Part model, mm, in its own coordinate system. A direction names the side the tool comes from. Round coordinates to 2 decimals unless told otherwise and drop trailing zeros. Loops run counter-clockwise (first coordinate to the right, second up) from the corner with the lowest first, then second, coordinate; pieces in that order, holes last. Notation, with made-up numbers: (4, 83) - (10, 83) arc R28 cw to (10, 103) - close; hole circle Ø4 at (-10, -18). An arc over 180 degrees is marked (long way). Write each question's results on one line, items separated by ' | '. Start each with the question number.
(1) Mould opens along X. For faces 4 (the face through (80.25, 2, -79)), 5 (the face through (58, 2, 80)), 6 (the face through (138.03, 2.18, -40.276)), 7 (the face through (46.263, 2, 0)) say: released by +X, released by -X, zero draft, split by the parting line, or undercut.
(2) Drill centre lines: L1, parallel to Z at x = 36, y = 1.55; L2, parallel to X at y = 2.9, z = -15; L3, parallel to Z at x = 105, y = 1.1. Where is each one in solid material? Low to high.
(3) Tool access for faces 1 (the face through (69, 2, 6)), 2 (the face through (153.27, 2.18, 57.43)), 3 (the face through (102, 2, -80)): list every direction of +Z, -Z, +X, -X, +Y, -Y with a clear straight run to the whole face (end or side of a thin tool).
(4) Cut at A-A, the plane x = 39. List the corners of the cut face in (y, z).
(5) Cut at B-B, the plane x = 112.5. List the corners of the cut face in (y, z), then the cut area to 3 significant figures.
(6) Flat gauge pins, fed straight in: P1, Ø2, axis at x = 49, y = 1.5, coming from the +Z side; P2, Ø1.3, axis at x = 10.5, y = 3, coming from the -Z side; P3, Ø1.5, axis at y = 2.5, z = -51.5, coming from the +X side. Where does each tip first touch, or does it go through?
(7) Cut at C-C, the plane y = 0.8. Give the number of separate pieces and of enclosed holes in the cut face, then the cut area to 3 significant figures.
from build123d import *

# Parameters (mm, degrees)
BOSS_EXTRUDE1_DEPTH = 4.3
CUT_EXTRUDE1_DEPTH  = 4.5
FILLET1_R           = 2
CUT_EXTRUDE2_DEPTH  = 10
SKETCH8_R           = 1.5
CUT_EXTRUDE3_DEPTH  = 10
SKETCH9_R           = 1.5
CUT_EXTRUDE4_DEPTH  = 10
CUT_EXTRUDE5_DEPTH  = 10
SKETCH11_R          = 1.5
CUT_EXTRUDE6_DEPTH  = 10
SKETCH12_R          = 1.5
CUT_EXTRUDE7_DEPTH  = 10
SKETCH7_R           = 1.5
SKETCH7_W           = 11
SKETCH7_H           = 3
CUT_EXTRUDE8_DEPTH  = 9
CUT_EXTRUDE9_DEPTH  = 10
SKETCH14_R          = 1.5
CUT_EXTRUDE10_DEPTH = 10
SKETCH15_W          = 5
SKETCH15_H          = 14
CUT_EXTRUDE11_DEPTH = 10
SKETCH16_R          = 1.5
CUT_EXTRUDE12_DEPTH = 10
SKETCH18_R          = 1.5
SKETCH18_W          = 28.4
SKETCH18_H          = 4
CUT_EXTRUDE13_DEPTH = 10


with BuildPart() as part:
    # Sketch2 → Boss-Extrude1 (new body)
    with BuildSketch(Plane(origin=(0, 0, 0), x_dir=(1, 0, 0), z_dir=(0, 1, 0))):
        Polygon((0, 0), (0, 65), (58, 65), (58, 95), (102, 95), (102, 65), (160, 65), (160, 0), align=None)
    extrude(amount=BOSS_EXTRUDE1_DEPTH)

    # Mirror1: part across plane


with BuildPart() as part_1:
    add(part.part)
    add(part.part.mirror(Plane(origin=(0, 4.3, 0), x_dir=(1, 0, 0), z_dir=(0, 0, -1))))

    # Sketch3 → Cut-Extrude1 (cut)
    with BuildSketch(Plane(origin=(0, 4.3, 0), x_dir=(1, 0, 0), z_dir=(0, 1, 0))):
        Polygon((160, 61.8), (160, -61.8), (157.155555556, -61.8), (120, -20), (80.012594795, 0), (80.012594795, 20), (120.012594795, 20), (157.156451185, 61.8), align=None)
    extrude(amount=-CUT_EXTRUDE1_DEPTH, mode=Mode.SUBTRACT)

    # Fillet1
    fillet1_edges = [part_1.edges().sort_by_distance(p)[0] for p in [
        (157.156451185, 2.15, -61.8),
        (157.155555556, 2.15, 61.8),
    ]]
    fillet(fillet1_edges, radius=FILLET1_R)

    # Sketch6 → Cut-Extrude2 (cut)
    with BuildSketch(Plane(origin=(0, 4.3, 0), x_dir=(1, 0, 0), z_dir=(0, 1, 0))):
        Polygon((9, -61.8), (49, -61.8), (49, -44.8), (43, -44.8), (43, -30.841820122), (15, -30.841820122), (15, -44.8), (9, -44.8), align=None)
        Polygon((9, 44.8), (15, 44.8), (15, 30.841820122), (43, 30.841820122), (43, 44.8), (49, 44.8), (49, 61.8), (9, 61.8), align=None)
    extrude(amount=-CUT_EXTRUDE2_DEPTH, mode=Mode.SUBTRACT)

    # Sketch8 → Cut-Extrude3 (cut)
    with BuildSketch(Plane(origin=(0, 4.3, 0), x_dir=(1, 0, 0), z_dir=(0, 1, 0))):
        with Locations(Location((6.5, 58.8, 0), (0, 0, 270))):
            Circle(SKETCH8_R)
        with Locations(Location((6.5, 48.8, 0), (0, 0, 270))):
            Circle(SKETCH8_R)
        with Locations(Location((51.5, 48.8, 0), (0, 0, 270))):
            Circle(SKETCH8_R)
        with Locations(Location((51.5, 58.8, 0), (0, 0, 270))):
            Circle(SKETCH8_R)
        with Locations(Location((6.5, -48.7, 0), (0, 0, 270))):
            Circle(SKETCH8_R)
        with Locations(Location((6.5, -58.7, 0), (0, 0, 270))):
            Circle(SKETCH8_R)
        with Locations(Location((51.5, -58.7, 0), (0, 0, 270))):
            Circle(SKETCH8_R)
        with Locations(Location((51.5, -48.8, 0), (0, 0, 270))):
            Circle(SKETCH8_R)
    extrude(amount=-CUT_EXTRUDE3_DEPTH, mode=Mode.SUBTRACT)

    # Sketch9 → Cut-Extrude4 (cut)
    with BuildSketch(Plane.XZ):
        with Locations(Location((94, 70.4, 0), (0, 0, 270))):
            Circle(SKETCH9_R)
        with Locations(Location((66, 78.4, 0), (0, 0, 270))):
            Circle(SKETCH9_R)
        with Locations(Location((66, -78.4, 0), (0, 0, 270))):
            Circle(SKETCH9_R)
        with Locations(Location((94, -86.4, 0), (0, 0, 270))):
            Circle(SKETCH9_R)
        with Locations(Location((94, 86.4, 0), (0, 0, 270))):
            Circle(SKETCH9_R)
        with Locations(Location((94, -70.4, 0), (0, 0, 270))):
            Circle(SKETCH9_R)
        with BuildLine():
            Line((75.75, 69.4), (75.75, 87.4))
            ThreePointArc((75.75, 87.4), (78, 89.65), (80.25, 87.4))
            Line((80.25, 87.4), (80.25, 69.4))
            ThreePointArc((80.25, 69.4), (78, 67.15), (75.75, 69.4))
        make_face()
        with BuildLine():
            Line((75.75, -87.4), (75.75, -70.4))
            ThreePointArc((75.75, -70.4), (78, -68.15), (80.25, -70.4))
            Line((80.25, -70.4), (80.25, -87.4))
            ThreePointArc((80.25, -87.4), (78, -89.65), (75.75, -87.4))
        make_face()
    extrude(amount=-CUT_EXTRUDE4_DEPTH, mode=Mode.SUBTRACT)

    # Sketch10 → Cut-Extrude5 (cut)
    with BuildSketch(Plane(origin=(0, 4.3, 0), x_dir=(1, 0, 0), z_dir=(0, 1, 0))):
        with BuildLine():
            Line((123.321819194, -23.737046593), (149.896372747, -53.633419341))
            Line((149.896372747, -53.633419341), (146.159326154, -56.955238535))
            Line((146.159326154, -56.955238535), (116.262953407, -23.321819194))
            ThreePointArc((116.262953407, -23.321819194), (120.29361011, -15.008628134), (123.321819194, -23.737046593))
        make_face()
    extrude(amount=-CUT_EXTRUDE5_DEPTH, mode=Mode.SUBTRACT)

    # Sketch11 → Cut-Extrude6 (cut)
    with BuildSketch(Plane.XZ):
        with BuildLine():
            Line((75, 31.031280577), (75, 15.031280577))
            ThreePointArc((75, 15.031280577), (77, 13.031280577), (79, 15.031280577))
            Line((79, 15.031280577), (79, 31.031280577))
            ThreePointArc((79, 31.031280577), (77, 33.031280577), (75, 31.031280577))
        make_face()
        with BuildLine():
            Line((75, -31.031280577), (75, -15.031280577))
            ThreePointArc((75, -15.031280577), (77, -13.031280577), (79, -15.031280577))
            Line((79, -15.031280577), (79, -31.031280577))
            ThreePointArc((79, -31.031280577), (77, -33.031280577), (75, -31.031280577))
        make_face()
        with Locations(Location((60, -31, 0), (0, 0, 270))):
            Circle(SKETCH11_R)
        with Locations(Location((60, 31, 0), (0, 0, 270))):
            Circle(SKETCH11_R)
        with Locations(Location((60, 15, 0), (0, 0, 270))):
            Circle(SKETCH11_R)
        with Locations(Location((60, -15, 0), (0, 0, 90))):
            Circle(SKETCH11_R)
    extrude(amount=-CUT_EXTRUDE6_DEPTH, mode=Mode.SUBTRACT)

    # Sketch12 → Cut-Extrude7 (cut)
    with BuildSketch(Plane(origin=(0, 0, 0), x_dir=(-1, 0, 0), z_dir=(0, -1, 0))):
        with BuildLine():
            Line((-50.262723036, 0), (-50.262723036, -8))
            ThreePointArc((-50.262723036, -8), (-48.262723036, -10), (-46.262723036, -8))
            Line((-46.262723036, -8), (-46.262723036, 0))
            Line((-46.262723036, 0), (-50.262723036, 0))
        make_face()
        with BuildLine():
            Line((-50.262723036, 8), (-50.262723036, 0))
            Line((-50.262723036, 0), (-46.262723036, 0))
            Line((-46.262723036, 0), (-46.262723036, 8))
            ThreePointArc((-46.262723036, 8), (-48.262723036, 10), (-50.262723036, 8))
        make_face()
        with Locations(Location((-32.262723036, -8, 0), (0, 0, 90))):
            Circle(SKETCH12_R)
        with Locations(Location((-32.262723036, 8, 0), (0, 0, 90))):
            Circle(SKETCH12_R)
    extrude(amount=-CUT_EXTRUDE7_DEPTH, mode=Mode.SUBTRACT)

    # Sketch7 → Cut-Extrude8 (cut)
    with BuildSketch(Plane(origin=(0, 4.3, 0), x_dir=(1, 0, 0), z_dir=(0, 1, 0))):
        with Locations(Location((60.012594795, -6.5, 0), (0, 0, 270))):
            Circle(SKETCH7_R)
        with Locations(Location((60.012594795, 6.5, 0), (0, 0, 270))):
            Circle(SKETCH7_R)
        with Locations(Location((86, 32.5, 0), (0, 0, 270))):
            Circle(SKETCH7_R)
        with Locations(Location((86, 45.5, 0), (0, 0, 270))):
            Circle(SKETCH7_R)
        with Locations((69.5, -7.5)):
            Rectangle(SKETCH7_W, SKETCH7_H)
        with Locations((69.5, 7.5)):
            Rectangle(SKETCH7_W, SKETCH7_H)
        with Locations((95.487405205, 31.5)):
            Rectangle(SKETCH7_W, SKETCH7_H)
        with Locations((95.487405205, 46.5)):
            Rectangle(SKETCH7_W, SKETCH7_H)
    extrude(amount=-CUT_EXTRUDE8_DEPTH, mode=Mode.SUBTRACT)

    # Sketch13 → Cut-Extrude9 (cut)
    with BuildSketch(Plane(origin=(0, 4.3, 0), x_dir=(1, 0, 0), z_dir=(0, 1, 0))):
        with BuildLine():
            ThreePointArc((63.5, 0), (65, -1.5), (66.5, 0))
            Line((66.5, 0), (63.5, 0))
        make_face()
        with BuildLine():
            Line((63.5, 0), (66.5, 0))
            ThreePointArc((66.5, 0), (65, 1.5), (63.5, 0))
        make_face()
        with BuildLine():
            ThreePointArc((73.5, 0), (75, -1.5), (76.5, 0))
            Line((76.5, 0), (73.5, 0))
        make_face()
        with BuildLine():
            Line((73.5, 0), (76.5, 0))
            ThreePointArc((76.5, 0), (75, 1.5), (73.5, 0))
        make_face()
    extrude(amount=-CUT_EXTRUDE9_DEPTH, mode=Mode.SUBTRACT)

    # Sketch14 → Cut-Extrude10 (cut)
    with BuildSketch(Plane(origin=(0, 4.3, 0), x_dir=(1, 0, 0), z_dir=(0, 1, 0))):
        with Locations(Location((57.5, 58.3, 0), (0, 0, 270))):
            Circle(SKETCH14_R)
        with Locations(Location((57.5, 21.3, 0), (0, 0, 270))):
            Circle(SKETCH14_R)
        with Locations(Location((85.370034901, -30.712866901, 0), (0, 0, 270))):
            Circle(SKETCH14_R)
        with Locations(Location((105.300950066, -53.135146462, 0), (0, 0, 270))):
            Circle(SKETCH14_R)
    extrude(amount=-CUT_EXTRUDE10_DEPTH, mode=Mode.SUBTRACT)

    # Sketch15 → Cut-Extrude11 (cut)
    with BuildSketch(Plane(origin=(0, 4.3, 0), x_dir=(1, 0, 0), z_dir=(0, 1, 0))):
        with Locations((48.5, 21)):
            Rectangle(SKETCH15_W, SKETCH15_H)
        with Locations((48.5, -21)):
            Rectangle(SKETCH15_W, SKETCH15_H)
    extrude(amount=-CUT_EXTRUDE11_DEPTH, mode=Mode.SUBTRACT)

    # Sketch16 → Cut-Extrude12 (cut)
    with BuildSketch(Plane(origin=(0, 4.3, 0), x_dir=(1, 0, 0), z_dir=(0, 1, 0))):
        with Locations(Location((89, -58.8, 0), (0, 0, 270))):
            Circle(SKETCH16_R)
        with Locations(Location((58, -58.8, 0), (0, 0, 270))):
            Circle(SKETCH16_R)
    extrude(amount=-CUT_EXTRUDE12_DEPTH, mode=Mode.SUBTRACT)

    # Sketch18 → Cut-Extrude13 (cut)
    with BuildSketch(Plane(origin=(0, 4.3, 0), x_dir=(1, 0, 0), z_dir=(0, 1, 0))):
        with Locations(Location((105, 50, 0), (0, 0, 270))):
            Circle(SKETCH18_R)
        with Locations(Location((120, 50, 0), (0, 0, 270))):
            Circle(SKETCH18_R)
        with Locations(Location((130.4, 50, 0), (0, 0, 270))):
            Circle(SKETCH18_R)
        with Locations((117.7, 58)):
            Rectangle(SKETCH18_W, SKETCH18_H)
        with Locations((117.7, 42)):
            Rectangle(SKETCH18_W, SKETCH18_H)
    extrude(amount=-CUT_EXTRUDE13_DEPTH, mode=Mode.SUBTRACT)


solid = part_1.part
A:
1) face 4: undercut | face 5: released by -X | face 6: released by +X | face 7: undercut
2) L1: -65 to -61.8, -30.84 to 30.84, 61.8 to 65 | L2: 0 to 46, 51 to 58.5, 61.5 to 75, 79 to 80.01 | L3: -65 to -60, -56 to -51.5, -48.5 to -44, -40 to -20, 12.5 to 51.67, 54.6 to 65
3) face 1: +Y, -Y | face 2: +X, +Y, -Y | face 3: -Z, +X, +Y, -Y
4) outline: (0, -65) - (4.3, -65) - (4.3, -61.8) - (0, -61.8) - close; (0, -30.84) - (4.3, -30.84) - (4.3, 30.84) - (0, 30.84) - close; (0, 61.8) - (4.3, 61.8) - (4.3, 65) - (0, 65) - close
5) outline: (0, -65) - (4.3, -65) - (4.3, -60) - (0, -60) - close; (0, -56) - (4.3, -56) - (4.3, -44) - (0, -44) - close; (0, -40) - (4.3, -40) - (4.3, -20) - (0, -20) - close; (0, 16.25) - (4.3, 16.25) - (4.3, 65) - (0, 65) - close | area: 369 mm2
6) P1: z = 65 | P2: z = -65 | P3: x = 148.67
7) separate pieces: 1 | enclosed holes: 50 | area: 15,300 mm2
